The listing builds one solid part. Answer for the finished solid, in the listing's coordinates (mm). Coordinates: 2 decimals unless noted, no trailing zeros. Loops run counter-clockwise (first coordinate to the right, second up) from the corner with the lowest first, then second, coordinate; pieces in that order, holes last. Notation, with made-up numbers: (-15.5, 55.5) - (31.5, 55.5) arc R10 ccw to (31.5, 59.5) - close; hole circle Ø3 at (4, 37.25). An arc over 180 degrees is marked (long way). Put each result on its own line as item: value.
Autodesk Inventor part; units mm, degrees
ref_plane "YZ Plane" through (0, 0, 0) normal (1, 0, 0) x (0, 1, 0)
ref_plane "XZ Plane" through (0, 0, 0) normal (0, 1, 0) x (-1, 0, 0)
ref_plane "XY Plane" through (0, 0, 0) normal (0, 0, 1) x (1, 0, 0)
sketch "Sketch1" plane through (0, 0, 0) normal (0, 0, 1) x (1, 0, 0)
  line L0 (5.3033, -5.3033) -> (0, 0) construction
  line L1 (0, 0) -> (-5.3033, -5.3033) construction
  line L2 (0, -10.6066) -> (10.6066, 0)
  line L3 (10.6066, 0) -> (5.7063, 11.8303)
  line L4 (5.7063, 11.8303) -> (-5.7063, 11.8303)
  line L5 (-5.7063, 11.8303) -> (-10.6066, 0)
  line L6 (-10.6066, 0) -> (0, -10.6066)
  line L7 (0, -10.6066) -> (0, 11.8303) construction
  dimension "d0" = 90
  dimension "d1" = 112.5
  dimension "d2" = 112.5
  dimension "d3" = 112.5
  dimension "d4" = 15
  dimension "d5" = 12.805
extrude "Extrusion1" add sketch "Sketch1" along normal blind 11
equation "\"d2\" = d1"
equation "\"d3\" = d1"
properties part number "Prisma-90" material "Glass"
1) The part is cut by section C-C (y = 10.5). Give the vertices of the cut face in (x, z), and give its area (3 significant figures).
Found:
outline: (-6.26, 0) - (6.26, 0) - (6.26, 11) - (-6.26, 11) - close
area: 138 mm^2
2) The part is cut by section B-B (x = -1.25). Give the vertices of the cut face in (y, z).
Found:
outline: (-9.36, 0) - (11.83, 0) - (11.83, 11) - (-9.36, 11) - close
3) The part is cut by section A-A (z = 3). Give the vertices of the cut face in (x, y).
Found:
outline: (-10.61, 0) - (0, -10.61) - (10.61, 0) - (5.71, 11.83) - (-5.71, 11.83) - close
4) For a pull along Y with two mould halves and no side action, classify faces 1 (the face through (0, 3, 0)), 2 (the face through (0, 11.83, 5)), 3 (the face through (-5.378, -5.229, 5.423)) as pulls with the +Y half, pulls with the -Y half, needs draft (parallel to the pull), parting line crosses it, or undercut.
Found:
face 1: needs draft
face 2: pulls with the +Y half
face 3: pulls with the -Y half
5) Straight lines are drawn through the part: L1, parallel to X at y = 3, z = 4.5; L2, parallel to X at y = -8, z = 2; L3, parallel to Y at x = 4.25, z = 8.25. For each, find the intervals that lie inside material, in ascending order. Write a range as [from, to].
Found:
L1: x = [-9.36, 9.36]
L2: x = [-2.61, 2.61]
L3: y = [-6.36, 11.83]
6) Each of these flat-tipped pins is pushed along its axis until it touches: pin 1 (3 mm diameter, centred on x = 4, z = 8.5, fed in from -Y); pin 2 (1.5 mm diameter, centred on x = -3, z = 8.5, fed in from -Y); pin 3 (3 mm diameter, centred on x = -3.5, z = 2.5, fed in from -Y). Where does it stop, or does it pass through?
Found:
pin 1: stops at y = -8.11
pin 2: stops at y = -8.36
pin 3: stops at y = -8.61
